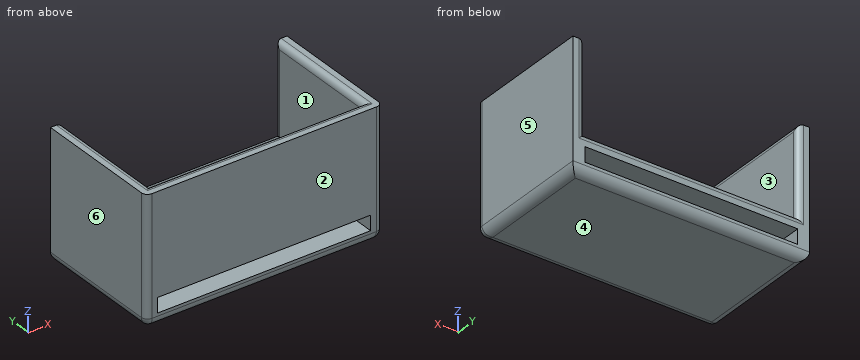
Autodesk Fusion 360 part; units mm, degrees
sketch "Skizze1" plane through (0, 0, 0) normal (0, 1, 0) x (1, 0, 0)
  line L0 (0, 0) -> (36, 0)
  line L1 (36, 0) -> (36, -15)
  line L2 (36, -15) -> (0, -15)
  line L3 (0, -15) -> (0, 0)
  line L4 (38, 2) -> (38, -17)
  line L5 (38, -17) -> (-2, -17)
  line L6 (-2, -17) -> (-2, 2)
  line L7 (-2, 2) -> (38, 2)
  line L8 (0, 2) -> (36, 2)
  line L9 (36, 2) -> (36, 4.5)
  line L10 (36, 4.5) -> (0, 4.5)
  line L11 (0, 4.5) -> (0, 2)
  line L12 (38, 2) -> (38, 6.5)
  line L13 (38, 6.5) -> (-2, 6.5)
  line L14 (-2, 6.5) -> (-2, 2)
  line L15 (0, -15) -> (-2, -15)
  line L16 (36, -15) -> (38, -15)
  dimension "d6" = 36
  dimension "d7" = 15
  dimension "d8" = 2
  dimension "d9" = 36
  dimension "d10" = 2.5
  dimension "d11" = 2
extrude "Extrusion1" add sketch "Skizze1" along normal blind 2 contours L0 L1 L2 L3
extrude "Extrusion2" add sketch "Skizze1" along normal blind 22 contours L0 L1 L3 L4 L6 L7 L8 L15 L16 | L7 L9 L10 L11 L12 L13 L14
fillet "Abrundung1" radius 1 6 edges at (0, 12, 15) (0, 22, 7.5) (18, 22, 0) (36, 22, 7.5) (36, 12, 15) (18, 2, 15)
fillet "Abrundung2" radius 1.5 4 edges at (18, 22, -6.5) (-2, 11, -6.5) (38, 11, -6.5) (18, 0, -6.5)
fillet "Abrundung3" radius 1 4 edges at (37.5607, 0.4393, -6.0607) (38, 0, 5) (-1.5607, 0.4393, -6.0607) (-2, 0, 5)
equation "width = 3.6 cm"
equation "height = 1.5 cm"
equation "depth = 2 cm"
equation "wall = 2 mm"
equation "space = 2.5 mm"
equation "d6 = width"
equation "d7 = height"
equation "d8 = wall"
equation "d9 = width"
equation "d10 = space"
equation "d11 = wall"
equation "d13 = wall"
equation "d15 = wall + depth"
Could you check a few things on this model? Use its own coordinates, in mm. Face numbers are marked on the shaded views. A direction names the side the tool comes from. Coordinates: 2 decimals unless noted, no trailing zeros. Loops run counter-clockwise (first coordinate to the right, second up) from the corner with the lowest first, then second, coordinate; pieces in that order, holes last.
1) Imagine slicing it at B-B (y = 10.5). List the corners of the cut face in (x, z) for me.
Reported:
outline: (-2, -5) arc R1.5 ccw to (-0.5, -6.5) - (36.5, -6.5) arc R1.5 ccw to (38, -5) - (38, 15) - (37, 15) arc R1 ccw to (36, 14) - (36, 0) - (0, 0) - (0, 14) arc R1 ccw to (-1, 15) - (-2, 15) - close; hole (0, -4.5) - (36, -4.5) - (36, -2) - (0, -2) - close
2) Please list where these lines run through material, in increasing order: line 1 along X through (y, z) = (2.25, 7.25); line 2 along Z through (x, y) = (10, 5); line 3 along Y through (x, z) = (24, 13.5).
Reported:
line 1: x = -2 to 0, 36 to 38
line 2: z = -6.5 to -4.5, -2 to 0
line 3: y = 0 to 2
3) Imagine slicing it at C-C (z = 0.5). List the corners of the cut face in (x, y) for me, and give its area (3 significant figures).
Reported:
outline: (-2, 1) arc R1 ccw to (-1, 0) - (37, 0) arc R1 ccw to (38, 1) - (38, 22) - (37, 22) arc R1 ccw to (36, 21) - (36, 2) - (0, 2) - (0, 21) arc R1 ccw to (-1, 22) - (-2, 22) - close
area: 159 mm2
4) Which directions (+Z, -Z, +X, -X, +Y, -Y) give clear straight access to the entire face, cutting with the end or side of a thin tool? Please do the marked faces 1 and 2.
Reported:
face 1: +Z, +Y
face 2: +Z, -Z, +X, -X, -Y
5) Will these pins go through, and if not, where does the flat tip stop? pin 1 Ø8 at (x, z) = (4, 10) entering from -Y; pin 2 Ø7 at (x, z) = (25, 7.5) entering from +Y; pin 3 Ø10 at (x, y) = (10.5, 8.5) entering from +Z; pin 4 Ø2 at (x, y) = (15, 2.5) entering from +Z.
Reported:
pin 1: stops at y = 0
pin 2: stops at y = 2
pin 3: stops at z = 0
pin 4: stops at z = 14.87
6) Imagine slicing it at A-A (x = 21.5). List the corners of the cut face in (y, z) for me, and give its area (3 significant figures).
Reported:
outline: (0, -5) arc R1.5 ccw to (1.5, -6.5) - (20.5, -6.5) arc R1.5 ccw to (22, -5) - (22, -4.5) - (0, -4.5) - close; (0, -2) - (22, -2) - (22, -1) arc R1 ccw to (21, 0) - (2, 0) - (2, 14) arc R1 ccw to (1, 15) - (0, 15) - close
area: 117 mm2
7) Thinking about a two-plate mould opening in X: for the marked faces 3, 4, 5 and 6, which applies, released by +X, released by -X, zero draft, split by the parting line, or undercut?
Reported:
face 3: undercut
face 4: zero draft
face 5: released by +X
face 6: released by -X
